The figure shows three views and two pictorial views of one solid part (mm, origin at its lowest corner). Answer the questions. A direction names the side the tool comes from. Give positions to 0.01 mm unless a question says otherwise; leave off trailing zeros. Loops run counter-clockwise (first coordinate to the right, second up) from the corner with the lowest first, then second, coordinate; pieces in that order, holes last. Notation, with made-up numbers: (36.25, -39.5) - (90.25, -39.5) arc R24 ccw to (90.25, -12.5) - close; hole circle Ø9 at (-9, 27.5). An arc over 180 degrees is marked (long way). Use CSV: the item, a comma, the result in double quotes.
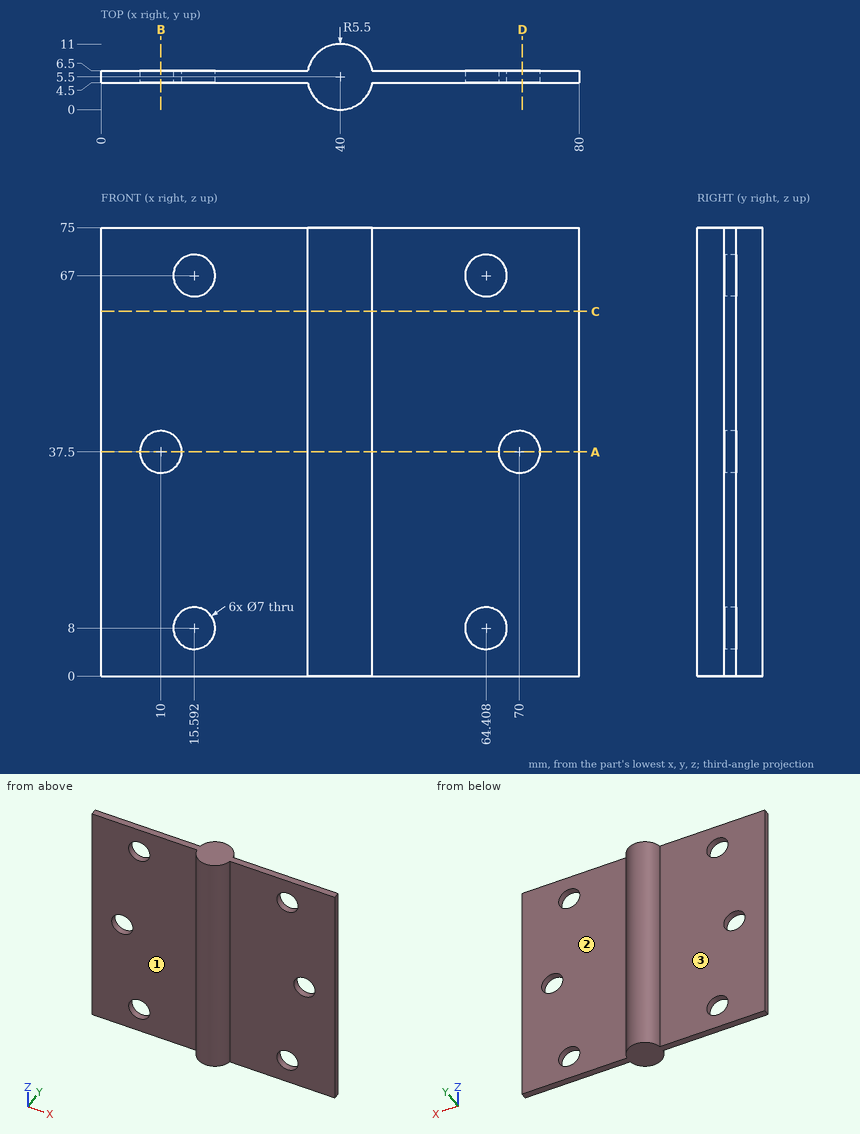
Item 1: A cutting plane is placed at A-A on z = 37.5. Determine the outline of the cut face in (x, y).
Determined:
outline,"(0, 4.5) - (6.5, 4.5) - (6.5, 6.5) - (0, 6.5) - close; (13.5, 4.5) - (34.59, 4.5) arc R5.5 ccw to (45.41, 4.5) - (66.5, 4.5) - (66.5, 6.5) - (45.41, 6.5) arc R5.5 ccw to (34.59, 6.5) - (13.5, 6.5) - close; (73.5, 4.5) - (80, 4.5) - (80, 6.5) - (73.5, 6.5) - close"
Item 2: A cutting plane is placed at B-B on x = 10. Determine the outline of the cut face in (y, z), and give its area (3 significant figures).
Determined:
outline,"(4.5, 0) - (6.5, 0) - (6.5, 34) - (4.5, 34) - close; (4.5, 41) - (6.5, 41) - (6.5, 75) - (4.5, 75) - close"
area,"136 mm²"
Item 3: A cutting plane is placed at D-D on x = 70.5. Determine the outline of the cut face in (y, z), and give its area (3 significant figures).
Determined:
outline,"(4.5, 0) - (6.5, 0) - (6.5, 34.04) - (4.5, 34.04) - close; (4.5, 40.96) - (6.5, 40.96) - (6.5, 75) - (4.5, 75) - close"
area,"136 mm²"
Item 4: A cutting plane is placed at C-C on z = 61. Determine the outline of the cut face in (x, y).
Determined:
outline,"(0, 4.5) - (34.59, 4.5) arc R5.5 ccw to (45.41, 4.5) - (80, 4.5) - (80, 6.5) - (45.41, 6.5) arc R5.5 ccw to (34.59, 6.5) - (0, 6.5) - close"
Item 5: For the marked faces 1, 2 and 3, determine the directions among +Z, -Z, +X, -X, +Y, -Y from which every point of the face is accessible in a straight line to the end or side of a thin tool.
Determined:
face 1,"+Z, -Z, -X, -Y"
face 2,"+Z, -Z, +X, +Y"
face 3,"+Z, -Z, -X, +Y"
Item 6: Given P1, Ø8, axis at x = 15.59, z = 67, coming from the +Y side; P2, Ø1, axis at x = 42.5, z = 49, coming from the +Y side; P3, Ø9, axis at x = 64.41, z = 67, coming from the -Y side, each flat-ended and moving along its own axis, determine where each tip first touches the part or whether it passes through.
Determined:
P1,"stops at y = 6.5"
P2,"stops at y = 10.62"
P3,"stops at y = 4.5"
Item 7: Find the intervals of material crossed by line 1 (Z direction, x = 70, y = 5.75); line 2 (X direction, y = 5, z = 38); line 3 (Y direction, x = 33, z = 6.5), in increasing order.
Determined:
line 1,"z = 0 to 34, 41 to 75"
line 2,"x = 0 to 6.54, 13.46 to 66.54, 73.46 to 80"
line 3,"y = 4.5 to 6.5"
